Check sheet for the drawn part. Datum: minimum x, y, z corner. Units: mm. Round coordinates to 2 decimals unless told otherwise and drop trailing zeros. Order: outer loops, then holes, each group sorted by start corner. A loop starts at its lowest first (then second) coordinate and runs counter-clockwise, first axis right, second up. Notation, with made-up numbers: (84, -34) -> (109, -34) arc R37 cw to (109, 3) -> close; hole circle Ø6 at (3.25, 0). An arc over 180 degrees is marked (long way). Write item = value, one per line. Start each with the question number.
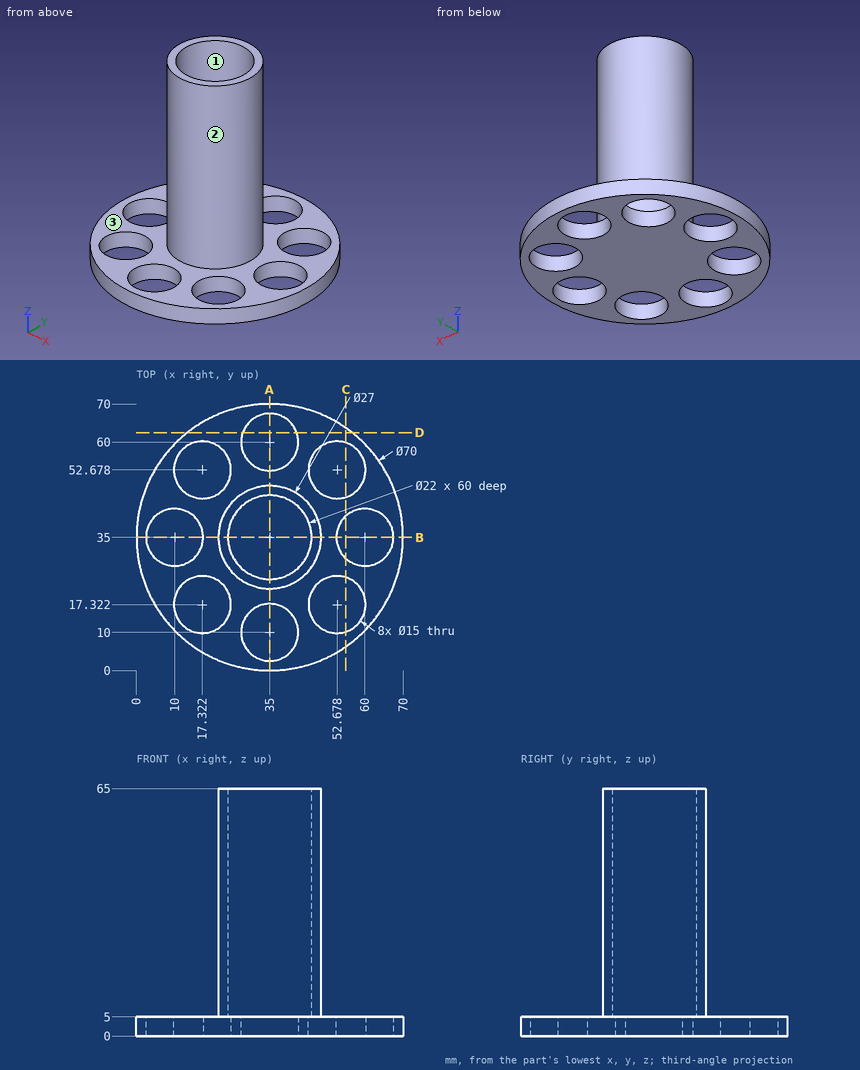
(1) Scan lines: line 1 along Y through (x, z) = (29.5, 3) (1 decimal); line 2 along Y through (x, z) = (51, 3.5); line 3 along Z through (x, y) = (16.5, 27). Record each from-to range of solid material in increasing order. Write a range as from..to.
(2) Cross-section at C-C (x = 55). Enter the section's corners in (y, z).
(3) Depth check by flat-ended pin: pin 1 (19.5 mm diameter, centred on x = 35, y = 60, fed in from -Z); pin 2 (20 mm diameter, centred on x = 35, y = 35, fed in from +Z); pin 3 (2 mm diameter, centred on y = 33, z = 33.5, fed in from +X); pin 4 (2 mm diameter, centred on x = 40, z = 37.5, fed in from -Y). Enter the tip coordinate at first touch or a pass-through.
(4) Cross-section at A-A (x = 35). Enter the section's corners in (y, z), and give its area (3 significant figures).
(5) Draft check along Y on the marked faces 1, 2 and 3. Enter one of: +Y half, -Y half, draft (parallel to the pull), parting line (faces both ways), or undercut.
(6) Cross-section at D-D (y = 62.5). Enter the section's corners in (x, z).
Outcome:
q1.line_1 = 0.4..4.9, 15.1..54.9, 65.1..69.6
q1.line_2 = 3.87..10.01, 24.63..45.37, 59.99..66.13
q1.line_3 = 0..5
q2.outline = (6.28, 0) -> (10.19, 0) -> (10.19, 5) -> (6.28, 5) -> close; (24.45, 0) -> (29.41, 0) -> (29.41, 5) -> (24.45, 5) -> close; (40.59, 0) -> (45.55, 0) -> (45.55, 5) -> (40.59, 5) -> close; (59.81, 0) -> (63.72, 0) -> (63.72, 5) -> (59.81, 5) -> close
q3.pin_1 = 0
q3.pin_2 = 5
q3.pin_3 = 48.46
q3.pin_4 = 22.11
q4.outline = (0, 0) -> (2.5, 0) -> (2.5, 5) -> (0, 5) -> close; (17.5, 0) -> (52.5, 0) -> (52.5, 5) -> (48.5, 5) -> (48.5, 65) -> (46, 65) -> (46, 5) -> (24, 5) -> (24, 65) -> (21.5, 65) -> (21.5, 5) -> (17.5, 5) -> close; (67.5, 0) -> (70, 0) -> (70, 5) -> (67.5, 5) -> close
q4.area = 500 mm^2
q5.face_1 = undercut
q5.face_2 = parting line
q5.face_3 = draft
q6.outline = (13.35, 0) -> (27.93, 0) -> (27.93, 5) -> (13.35, 5) -> close; (42.07, 0) -> (56.65, 0) -> (56.65, 5) -> (42.07, 5) -> close
